Check sheet for the modelled part. Datum: model origin and axes. Units: mm. Coordinates: 2 decimals unless noted, no trailing zeros. Loops run counter-clockwise (first coordinate to the right, second up) from the corner with the lowest first, then second, coordinate; pieces in that order, holes last.
```python
from build123d import *

# Parameters (mm, degrees)
SKICA1_W                 = 340
SKICA1_H                 = 380
SKICA1_R                 = 2.5
P_IDAT_VYSUNUT_M1_DEPTH  = 2
SKICA2_R                 = 1.650000196
SKICA2_R_2               = 1.649999612
SKICA2_R_3               = 4.150000099
SKICA2_R_4               = 4.149999924
SKICA2_R_5               = 4.149999975
SKICA2_R_6               = 4.150000026
SKICA2_R_7               = 12
ODEBRAT_VYSUNUT_M1_DEPTH = 2


with BuildPart() as part:
    # Skica1 → Přidat vysunutím1 (new body)
    with BuildSketch(Plane(origin=(0, 0, 0), x_dir=(1, 0, 0), z_dir=(0, 1, 0))):
        Rectangle(SKICA1_W, SKICA1_H)
        with Locations(Location((-160, 180, 0), (0, 0, 270))):
            Circle(SKICA1_R, mode=Mode.SUBTRACT)
        with Locations(Location((-54, 180, 0), (0, 0, 270))):
            Circle(SKICA1_R, mode=Mode.SUBTRACT)
        with Locations(Location((52, 180, 0), (0, 0, 270))):
            Circle(SKICA1_R, mode=Mode.SUBTRACT)
        with Locations(Location((158, 180, 0), (0, 0, 270))):
            Circle(SKICA1_R, mode=Mode.SUBTRACT)
        with Locations(Location((-54, -180, 0), (0, 0, 270))):
            Circle(SKICA1_R, mode=Mode.SUBTRACT)
        with Locations(Location((52, -180, 0), (0, 0, 270))):
            Circle(SKICA1_R, mode=Mode.SUBTRACT)
        with Locations(Location((158, -180, 0), (0, 0, 270))):
            Circle(SKICA1_R, mode=Mode.SUBTRACT)
        with Locations(Location((-160, -180, 0), (0, 0, 270))):
            Circle(SKICA1_R, mode=Mode.SUBTRACT)
    extrude(amount=P_IDAT_VYSUNUT_M1_DEPTH)

    # Skica2 → Odebrat vysunutím1 (cut)
    with BuildSketch(Plane.XZ):
        with Locations(Location((15.500000611, 162.999999867, 0), (0, 0, 270))):
            Circle(SKICA2_R)
        with Locations(Location((-15.499999389, 162.999999867, 0), (0, 0, 270))):
            Circle(SKICA2_R)
        with Locations(Location((-15.499999389, 131.999999867, 0), (0, 0, 270))):
            Circle(SKICA2_R)
        with Locations(Location((15.500000611, 131.999999867, 0), (0, 0, 270))):
            Circle(SKICA2_R)
        with Locations(Location((15.499999439, -162.999999266, 0), (0, 0, 270))):
            Circle(SKICA2_R_2)
        with Locations(Location((-15.500000561, -162.999999266, 0), (0, 0, 270))):
            Circle(SKICA2_R_2)
        with Locations(Location((-15.500000561, -131.999999266, 0), (0, 0, 270))):
            Circle(SKICA2_R_2)
        with Locations(Location((15.499999439, -131.999999266, 0), (0, 0, 270))):
            Circle(SKICA2_R_2)
        with Locations(Location((96.499999368, -147.499999005, 0), (0, 0, 270))):
            Circle(SKICA2_R_3)
        with Locations(Location((-96.499999659, -147.499999158, 0), (0, 0, 270))):
            Circle(SKICA2_R_4)
        with Locations(Location((-96.500017816, 147.499999068, 0), (0, 0, 270))):
            Circle(SKICA2_R_5)
        with Locations(Location((96.499999563, 147.499999035, 0), (0, 0, 270))):
            Circle(SKICA2_R_6)
        with Locations(Location((0, -147.499999158, 0), (0, 0, 270))):
            Circle(SKICA2_R_7)
        with Locations(Location((0, 147.499999035, 0), (0, 0, 270))):
            Circle(SKICA2_R_7)
    extrude(amount=-ODEBRAT_VYSUNUT_M1_DEPTH, mode=Mode.SUBTRACT)


solid = part.part
```
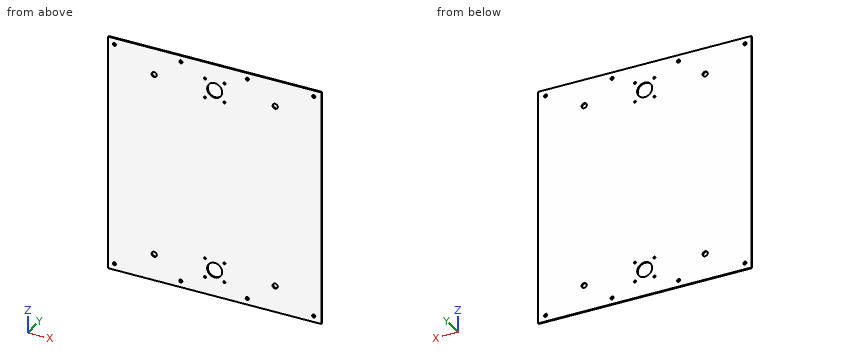
1) Section check A-A on x = 0. Enter the section's corners in (y, z).
Answer sheet:
outline: (0, -190) - (2, -190) - (2, -159.5) - (0, -159.5) - close; (0, -135.5) - (2, -135.5) - (2, 135.5) - (0, 135.5) - close; (0, 159.5) - (2, 159.5) - (2, 190) - (0, 190) - close
2) Depth check by flat-ended pin: pin 1 (2 mm diameter, centred on x = -15.5, z = -163, fed in from +Y). Enter the tip coordinate at first touch or a pass-through.
Answer sheet:
pin 1: passes through
3) Scan lines: line 1 (X direction, y = 1.05, z = -180); line 2 (X direction, y = 1.35, z = -147.5); line 3 (Z direction, x = -56, y = 0.75). Record each from-to range of solid material in increasing order.
Answer sheet:
line 1: x = -170 to -162.5, -157.5 to -56.5, -51.5 to 49.5, 54.5 to 155.5, 160.5 to 170
line 2: x = -170 to -100.65, -92.35 to -12, 12 to 92.35, 100.65 to 170
line 3: z = -190 to -181.5, -178.5 to 178.5, 181.5 to 190
